Read the model definition and answer for the solid it produces. Units are mm, in the model's axes. Face numbers are marked on the shaded views. A direction names the side the tool comes from. Coordinates: 2 decimals unless noted, no trailing zeros. Loops run counter-clockwise (first coordinate to the right, second up) from the corner with the lowest first, then second, coordinate; pieces in that order, holes last.
from build123d import *

# Parameters (mm, degrees)
SKETCH1_R           = 10.16
SKETCH1_R_2         = 9.25
BOSS_EXTRUDE1_DEPTH = 12
BOSS_EXTRUDE3_DEPTH = 11
BOSS_EXTRUDE4_DEPTH = 12


with BuildPart() as part:
    # Sketch1 → Boss-Extrude1 (new body)
    with BuildSketch(Plane(origin=(0, 0, 0), x_dir=(1, 0, 0), z_dir=(0, 1, 0))):
        Circle(SKETCH1_R)
        Circle(SKETCH1_R_2, mode=Mode.SUBTRACT)
    extrude(amount=BOSS_EXTRUDE1_DEPTH)

    # Sketch3 → Boss-Extrude3 (add, symmetric)
    with BuildSketch(Plane(origin=(0, 6, 0), x_dir=(-1, 0, 0), z_dir=(0, -1, 0))):
        with BuildLine():
            Line((5.212386984, 14.320915541), (3.474924656, 9.547277027))
            ThreePointArc((3.474924656, 9.547277027), (1.764265485, 10.005646771), (0, 10.16))
            Line((0, 10.16), (0, 15.24))
            ThreePointArc((0, 15.24), (2.646398228, 15.008470156), (5.212386984, 14.320915541))
        make_face()
        with BuildLine():
            Line((10.776307345, 10.776307345), (7.184204897, 7.184204897))
            ThreePointArc((7.184204897, 7.184204897), (8.32258477, 5.827536593), (9.208087116, 4.293801539))
            Line((9.208087116, 4.293801539), (13.812130674, 6.440702309))
            ThreePointArc((13.812130674, 6.440702309), (12.483877155, 8.74130489), (10.776307345, 10.776307345))
        make_face()
        with BuildLine():
            Line((15.24, 0), (10.16, 0))
            ThreePointArc((10.16, 0), (10.005646771, -1.764265485), (9.547277027, -3.474924656))
            Line((9.547277027, -3.474924656), (14.320915541, -5.212386984))
            ThreePointArc((14.320915541, -5.212386984), (15.008470156, -2.646398228), (15.24, 0))
        make_face()
        with BuildLine():
            Line((10.776307345, -10.776307345), (7.184204897, -7.184204897))
            ThreePointArc((7.184204897, -7.184204897), (5.827536593, -8.32258477), (4.293801539, -9.208087116))
            Line((4.293801539, -9.208087116), (6.440702309, -13.812130674))
            ThreePointArc((6.440702309, -13.812130674), (8.74130489, -12.483877155), (10.776307345, -10.776307345))
        make_face()
        with BuildLine():
            Line((0, -15.24), (0, -10.16))
            ThreePointArc((0, -10.16), (-1.764265485, -10.005646771), (-3.474924656, -9.547277027))
            Line((-3.474924656, -9.547277027), (-5.212386984, -14.320915541))
            ThreePointArc((-5.212386984, -14.320915541), (-2.646398228, -15.008470156), (0, -15.24))
        make_face()
        with BuildLine():
            Line((-10.776307345, -10.776307345), (-7.184204897, -7.184204897))
            ThreePointArc((-7.184204897, -7.184204897), (-8.32258477, -5.827536593), (-9.208087116, -4.293801539))
            Line((-9.208087116, -4.293801539), (-13.812130674, -6.440702309))
            ThreePointArc((-13.812130674, -6.440702309), (-12.483877155, -8.74130489), (-10.776307345, -10.776307345))
        make_face()
        with BuildLine():
            Line((-15.24, 0), (-10.16, 0))
            ThreePointArc((-10.16, 0), (-10.005646771, 1.764265485), (-9.547277027, 3.474924656))
            Line((-9.547277027, 3.474924656), (-14.320915541, 5.212386984))
            ThreePointArc((-14.320915541, 5.212386984), (-15.008470156, 2.646398228), (-15.24, 0))
        make_face()
        with BuildLine():
            Line((-10.776307345, 10.776307345), (-7.184204897, 7.184204897))
            ThreePointArc((-7.184204897, 7.184204897), (-5.827536593, 8.32258477), (-4.293801539, 9.208087116))
            Line((-4.293801539, 9.208087116), (-6.440702309, 13.812130674))
            ThreePointArc((-6.440702309, 13.812130674), (-8.74130489, 12.483877155), (-10.776307345, 10.776307345))
        make_face()
    extrude(amount=BOSS_EXTRUDE3_DEPTH, both=True)

    # Sketch4 → Boss-Extrude4 (add)
    with BuildSketch(Plane.XZ):
        with BuildLine():
            Line((-4, -4.75), (-4, -6.620469825))
            Line((-4, -6.620469825), (-1.5, -6.620469825))
            Line((-1.5, -6.620469825), (-1.5, -8.620469825))
            Line((-1.5, -8.620469825), (-1.5, -9.127568132))
            ThreePointArc((-1.5, -9.127568132), (0, -9.25), (1.5, -9.127568132))
            Line((1.5, -9.127568132), (1.5, -8.620469825))
            Line((1.5, -8.620469825), (1.5, -6.620469825))
            Line((1.5, -6.620469825), (4, -6.620469825))
            Line((4, -6.620469825), (4, -4.75))
            Line((4, -4.75), (-4, -4.75))
        make_face()
    extrude(amount=-BOSS_EXTRUDE4_DEPTH)


solid = part.part
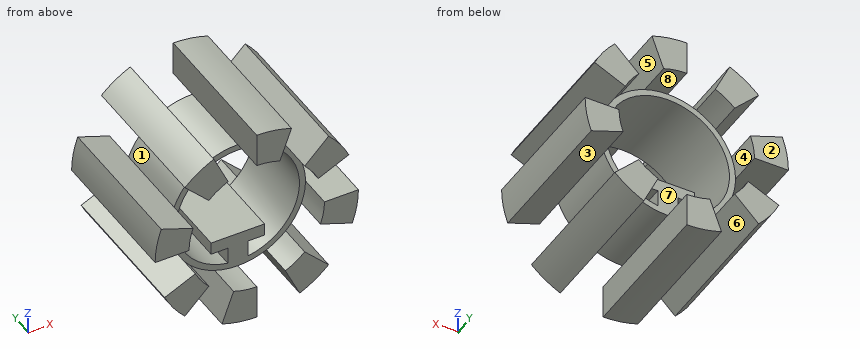
Q1. Which of the six approach directions +Z, -Z, +X, -X, +Y, -Y give full straight-line access (tool end or side, diameter ignored) to the marked faces 5, 6, 7 and 8?
Findings below:
face 5: +Y, -Y
face 6: -Z, +Y, -Y
face 7: +Y
face 8: -Z, +Y
Q2. A cutting plane is placed at C-C (x = -3). Give the vertices of the cut face in (y, z).
Findings below:
outline: (-5, -14.94) - (17, -14.94) - (17, -9.71) - (12, -9.71) - (12, -8.75) - (0, -8.75) - (0, -9.71) - (-5, -9.71) - close; (0, -6.62) - (12, -6.62) - (12, -4.75) - (0, -4.75) - close; (0, 8.75) - (12, 8.75) - (12, 9.71) - (0, 9.71) - close
Q3. A cutting plane is placed at B-B (z = -6). Give the vertices of the cut face in (x, y), then the cut area to 3 significant figures.
Findings below:
outline: (-12.87, -5) - (-8.2, -5) - (-8.2, 0) - (-7.04, 0) - (-7.04, 12) - (-8.2, 12) - (-8.2, 17) - (-12.87, 17) - close; (-4, 0) - (4, 0) - (4, 12) - (-4, 12) - close; (7.04, 0) - (8.2, 0) - (8.2, 12) - (7.04, 12) - close
area: 227 mm2
Q4. Flat-ended cylindrical pins translate along their axes: pin 1 Ø6 at (y, z) = (1, 2.5) entering from -X; pin 2 Ø2.5 at (x, y) = (-13.5, 4.5) entering from -Z; pin 3 Ø4 at (y, z) = (5, 12) entering from -X; pin 4 Ø1.5 at (x, y) = (-3.5, 7.5) entering from -Z. Find the tip coordinate at first contact, or state that the pin passes through.
Findings below:
pin 1: stops at x = -15.24
pin 2: stops at z = -9.07
pin 3: stops at x = -10.78
pin 4: stops at z = -14.99
Q5. Determine the mould class of the marked faces 1, 2, 3 and 4 for opening direction X: +X half, -X half, draft (parallel to the pull), parting line (faces both ways), or undercut.
Findings below:
face 1: undercut
face 2: draft
face 3: undercut
face 4: +X half
Q6. A cutting plane is placed at A-A (x = 1). Give the vertices of the cut face in (y, z), then the cut area to 3 significant figures.
Findings below:
outline: (-5, 10.11) - (0, 10.11) - (0, 9.2) - (12, 9.2) - (12, 10.11) - (17, 10.11) - (17, 15.21) - (-5, 15.21) - close; (0, -10.11) - (12, -10.11) - (12, -4.75) - (0, -4.75) - close
area: 187 mm2
Q7. Straight lines are drawn through the part: probe 1 along X at (y, z) = (8.25, -8); probe 2 along X at (y, z) = (15.75, 11); probe 3 along X at (y, z) = (13.75, -8.5). For each, find the intervals that lie inside material, in ascending order.
Findings below:
probe 1: x = -12.97 to -8, -6.26 to -4.64, -1.5 to 1.5, 4.64 to 8
probe 2: x = -10.55 to -5.13, 0 to 4
probe 3: x = -12.65 to -8.5, 5.57 to 8.5
Q8. A cutting plane is placed at D-D (z = 13). Give the vertices of the cut face in (x, y), then the cut area to 3 significant figures.
Findings below:
outline: (-7.95, -5) - (-6.06, -5) - (-6.06, 17) - (-7.95, 17) - close; (0, -5) - (4.73, -5) - (4.73, 17) - (0, 17) - close
area: 146 mm2
